Here's how the part is built. I have some questions about the finished solid (model axes, mm). Face numbers are marked on the shaded views. A direction names the side the tool comes from. Give positions to 0.01 mm unless a question says otherwise; leave off trailing zeros. Loops run counter-clockwise (first coordinate to the right, second up) from the corner with the lowest first, then second, coordinate; pieces in that order, holes last.
Q1. Will these pins go through, and if not, where does the flat tip stop? P1, Ø1.5, axis at y = -34.5, z = 77, coming from the +X side; P2, Ø8, axis at y = 90, z = 65, coming from the -X side.
Q2. For the marked faces 1 and 2, which set-ups out of +Z, -Z, +X, -X, +Y, -Y let a thin tool reach every point of the face, with its end or its side?
Q3. If we section it at C-C (x = 91): Please give me the cut outline in (y, z).
Q4. If we section it at A-A (z = 0): Please give me the cut outline in (x, y).
Q5. We'd pull the mould along X, two halves only. Please class the marked faces 3, 4 and 5: +X half, -X half, draft (parallel to the pull), parting line (faces both ways), or undercut.
Q6. I need wall thicknesses on line 1 (Y direction, x = 0.95, z = 65); line 2 (Z direction, x = 9.5, y = 0); line 3 (Y direction, x = 84.5, z = 22.5). Which ranges of each line are inside material? Lowest first, please.
Q7. If we section it at B-B (y = -74): Please give me the cut outline in (x, z).
Q8. If we section it at D-D (z = 29): Please give me the cut outline in (x, y).
from build123d import *

# Parameters (mm, degrees)
SKETCH_1_W          = 200
SKETCH_1_H          = 209
EXTRUDE_1_DEPTH     = 100
SHELL_1_T           = 2
CUT_EXTRUDE_1_REACH = 177.842
SKETCH_2_W          = 170
SKETCH_2_H          = 179
CUT_EXTRUDE_2_REACH = 177.842
SKETCH_3_R          = 2.5
CUT_EXTRUDE_3_REACH = 177.842
SKETCH_4_R          = 5


with BuildPart() as part:
    # 草图1 → 凸台-拉伸1 (new body)
    with BuildSketch(Plane(origin=(0, 0, 0), x_dir=(0, 0, -1), z_dir=(1, 0, 0))):
        Rectangle(SKETCH_1_W, SKETCH_1_H)
    extrude(amount=EXTRUDE_1_DEPTH)

    # 抽壳1 (no face opened: a closed hollow body)
    add(offset(amount=-SHELL_1_T, mode=Mode.PRIVATE), mode=Mode.SUBTRACT)

    # 草图2 → 切除-拉伸1 (cut, up to next)
    with BuildSketch(Plane(origin=(100, 0, 0), x_dir=(0, 0, -1), z_dir=(1, 0, 0)), mode=Mode.PRIVATE) as cut_extrude_1_sk1:
        Rectangle(SKETCH_2_W, SKETCH_2_H)
    cut_extrude_1_tool1 = extrude(cut_extrude_1_sk1.sketch, amount=-CUT_EXTRUDE_1_REACH, mode=Mode.PRIVATE) & part.part
    add(cut_extrude_1_tool1.solids().sort_by_distance((100, 0, 0))[0], mode=Mode.SUBTRACT)

    # 草图3 → 切除-拉伸2 (cut, up to next)
    with BuildSketch(Plane(origin=(100, 0, 0), x_dir=(0, 0, -1), z_dir=(1, 0, 0)), mode=Mode.PRIVATE) as cut_extrude_2_sk1:
        with Locations((0, 96.5)):
            Circle(SKETCH_3_R)
    cut_extrude_2_tool1 = extrude(cut_extrude_2_sk1.sketch, amount=-CUT_EXTRUDE_2_REACH, mode=Mode.PRIVATE) & part.part
    # 草图3 → 切除-拉伸2 (cut, up to next)
    with BuildSketch(Plane(origin=(100, 0, 0), x_dir=(0, 0, -1), z_dir=(1, 0, 0)), mode=Mode.PRIVATE) as cut_extrude_2_sk2:
        with Locations((-92, 0)):
            Circle(SKETCH_3_R)
    cut_extrude_2_tool2 = extrude(cut_extrude_2_sk2.sketch, amount=-CUT_EXTRUDE_2_REACH, mode=Mode.PRIVATE) & part.part
    # 草图3 → 切除-拉伸2 (cut, up to next)
    with BuildSketch(Plane(origin=(100, 0, 0), x_dir=(0, 0, -1), z_dir=(1, 0, 0)), mode=Mode.PRIVATE) as cut_extrude_2_sk3:
        with Locations((0, -96.5)):
            Circle(SKETCH_3_R)
    cut_extrude_2_tool3 = extrude(cut_extrude_2_sk3.sketch, amount=-CUT_EXTRUDE_2_REACH, mode=Mode.PRIVATE) & part.part
    # 草图3 → 切除-拉伸2 (cut, up to next)
    with BuildSketch(Plane(origin=(100, 0, 0), x_dir=(0, 0, -1), z_dir=(1, 0, 0)), mode=Mode.PRIVATE) as cut_extrude_2_sk4:
        with Locations((92, 0)):
            Circle(SKETCH_3_R)
    cut_extrude_2_tool4 = extrude(cut_extrude_2_sk4.sketch, amount=-CUT_EXTRUDE_2_REACH, mode=Mode.PRIVATE) & part.part
    add(cut_extrude_2_tool1.solids().sort_by_distance((100, 96.5, 0))[0], mode=Mode.SUBTRACT)
    add(cut_extrude_2_tool2.solids().sort_by_distance((100, 0, 92))[0], mode=Mode.SUBTRACT)
    add(cut_extrude_2_tool3.solids().sort_by_distance((100, -96.5, 0))[0], mode=Mode.SUBTRACT)
    add(cut_extrude_2_tool4.solids().sort_by_distance((100, 0, -92))[0], mode=Mode.SUBTRACT)

    # 草图4 → 切除-拉伸3 (cut, up to next)
    with BuildSketch(Plane.ZY, mode=Mode.PRIVATE) as cut_extrude_3_sk1:
        with Locations((-65, 90)):
            Circle(SKETCH_4_R)
    cut_extrude_3_tool1 = extrude(cut_extrude_3_sk1.sketch, amount=-CUT_EXTRUDE_3_REACH, mode=Mode.PRIVATE) & part.part
    # 草图4 → 切除-拉伸3 (cut, up to next)
    with BuildSketch(Plane.ZY, mode=Mode.PRIVATE) as cut_extrude_3_sk2:
        with Locations(Location((65, 90, 0), (0, 0, 180))):
            Circle(SKETCH_4_R)
    cut_extrude_3_tool2 = extrude(cut_extrude_3_sk2.sketch, amount=-CUT_EXTRUDE_3_REACH, mode=Mode.PRIVATE) & part.part
    # 草图4 → 切除-拉伸3 (cut, up to next)
    with BuildSketch(Plane.ZY, mode=Mode.PRIVATE) as cut_extrude_3_sk3:
        with Locations(Location((-65, -90, 0), (0, 0, 180))):
            Circle(SKETCH_4_R)
    cut_extrude_3_tool3 = extrude(cut_extrude_3_sk3.sketch, amount=-CUT_EXTRUDE_3_REACH, mode=Mode.PRIVATE) & part.part
    # 草图4 → 切除-拉伸3 (cut, up to next)
    with BuildSketch(Plane.ZY, mode=Mode.PRIVATE) as cut_extrude_3_sk4:
        with Locations((65, -90)):
            Circle(SKETCH_4_R)
    cut_extrude_3_tool4 = extrude(cut_extrude_3_sk4.sketch, amount=-CUT_EXTRUDE_3_REACH, mode=Mode.PRIVATE) & part.part
    add(cut_extrude_3_tool1.solids().sort_by_distance((0, 90, -65))[0], mode=Mode.SUBTRACT)
    add(cut_extrude_3_tool2.solids().sort_by_distance((0, 90, 65))[0], mode=Mode.SUBTRACT)
    add(cut_extrude_3_tool3.solids().sort_by_distance((0, -90, -65))[0], mode=Mode.SUBTRACT)
    add(cut_extrude_3_tool4.solids().sort_by_distance((0, -90, 65))[0], mode=Mode.SUBTRACT)


solid = part.part
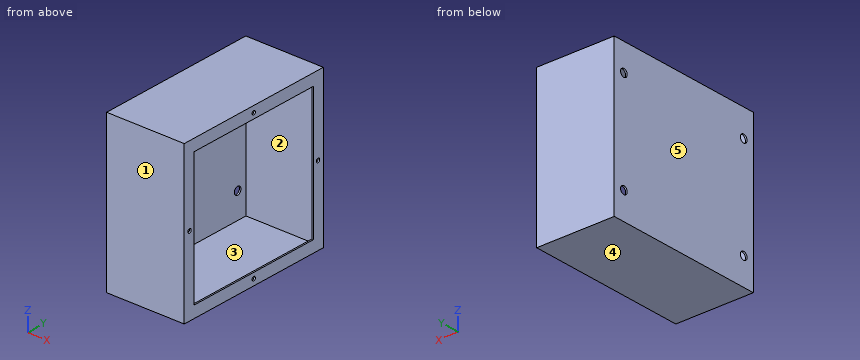
Check sheet entries:
1. P1: stops at x = 2
1. P2: stops at x = 98
2. face 1: +Z, -Z, +X, -X, -Y
2. face 2: none
3. outline: (-104.5, -100) - (104.5, -100) - (104.5, 100) - (-104.5, 100) - close; hole (-102.5, -98) - (102.5, -98) - (102.5, 98) - (-102.5, 98) - close
4. outline: (0, -104.5) - (100, -104.5) - (100, -99) - (98, -99) - (98, -102.5) - (2, -102.5) - (2, 102.5) - (98, 102.5) - (98, 99) - (100, 99) - (100, 104.5) - (0, 104.5) - close; (98, -94) - (100, -94) - (100, -89.5) - (98, -89.5) - close; (98, 89.5) - (100, 89.5) - (100, 94) - (98, 94) - close
5. face 3: undercut
5. face 4: draft
5. face 5: -X half
6. line 1: y = -104.5 to -95, -85 to 85, 95 to 104.5
6. line 2: z = -100 to -98, 98 to 100
6. line 3: y = -104.5 to -102.5, 102.5 to 104.5
7. outline: (0, -100) - (100, -100) - (100, -85) - (98, -85) - (98, -98) - (2, -98) - (2, 98) - (98, 98) - (98, 85) - (100, 85) - (100, 100) - (0, 100) - close
8. outline: (0, -104.5) - (100, -104.5) - (100, -89.5) - (98, -89.5) - (98, -102.5) - (2, -102.5) - (2, 102.5) - (98, 102.5) - (98, 89.5) - (100, 89.5) - (100, 104.5) - (0, 104.5) - close
